from build123d import *

# Parameters (mm, degrees)
SKETCH1_R           = 37.5
SKETCH1_R_2         = 35
BOSS_EXTRUDE1_DEPTH = 40
BOSS_EXTRUDE1_TAPER = 2
CUT_EXTRUDE1_DEPTH  = 40
CIRPATTERN1_COUNT   = 10
CUT_EXTRUDE2_DEPTH  = 40
CIRPATTERN2_COUNT   = 7
CIRPATTERN2_ANGLE   = 309


with BuildPart() as part:
    # Sketch1 → Boss-Extrude1 (new body)
    with BuildSketch(Plane(origin=(0, 0, 0), x_dir=(1, 0, 0), z_dir=(0, 1, 0))):
        Circle(SKETCH1_R)
        Circle(SKETCH1_R_2, mode=Mode.SUBTRACT)
    extrude(amount=BOSS_EXTRUDE1_DEPTH, taper=BOSS_EXTRUDE1_TAPER)

    # Sketch2 → Cut-Extrude1 (cut)
    with BuildSketch(Plane(origin=(0, 0, 0), x_dir=(0, 0, -1), z_dir=(1, 0, 0))):
        with BuildLine():
            Line((-3.5, 35.795316604), (-7.534748759, 33.202081775))
            Line((-7.534748759, 33.202081775), (-4.593988586, 28.626627084))
            Line((-4.593988586, 28.626627084), (0, 25.914355347))
            Line((0, 25.914355347), (4.219955288, 28.626627084))
            Line((4.219955288, 28.626627084), (6.92128469, 33.202081775))
            Line((6.92128469, 33.202081775), (3.5, 35.795316604))
            ThreePointArc((3.5, 35.795316604), (0, 39.295316604), (-3.5, 35.795316604))
        make_face()
    cut_extrude1 = extrude(amount=-CUT_EXTRUDE1_DEPTH, mode=Mode.SUBTRACT)

    # CirPattern1: Cut-Extrude1 ×10 about axis
    cirpattern1_axis = Axis((0, 0, 0), (0, 1, 0))
    for i in range(1, CIRPATTERN1_COUNT):
        add(cut_extrude1.rotate(cirpattern1_axis, i * 360 / CIRPATTERN1_COUNT), mode=Mode.SUBTRACT)

    # Sketch3 → Cut-Extrude2 (cut)
    with BuildSketch(Plane(origin=(0, 0, 0), x_dir=(0, 0, -1), z_dir=(1, 0, 0))):
        Polygon((0, 21.378578538), (-5.541834778, 18.44293311), (0, 6.63639335), (5.541834778, 18.44293311), align=None)
    cut_extrude2 = extrude(amount=-CUT_EXTRUDE2_DEPTH, mode=Mode.SUBTRACT)

    # CirPattern2: Cut-Extrude2 ×7 about axis
    cirpattern2_axis = Axis((0, 0, 0), (0, 1, 0))
    for i in range(1, CIRPATTERN2_COUNT):
        add(cut_extrude2.rotate(cirpattern2_axis, i * CIRPATTERN2_ANGLE / (CIRPATTERN2_COUNT - 1)), mode=Mode.SUBTRACT)


solid = part.part
The model under review builds one solid part; all positions refer to its coordinate system, in mm. A direction names the side the tool comes from. Round coordinates to 2 decimals unless told otherwise and drop trailing zeros. Loops run counter-clockwise (first coordinate to the right, second up) from the corner with the lowest first, then second, coordinate; pieces in that order, holes last. Notation, with made-up numbers: (86, -1.75) -> (133, -1.75) arc R19 cw to (133, 14.25) -> close; hole circle Ø9 at (-37.5, 16). An arc over 180 degrees is marked (long way). Write item = value, one per line. Start each with the question number.
Item 1: To check wall thickness, follow L1, parallel to Z at x = 11, y = 24.5; L2, parallel to Z at x = -2, y = 6; L3, parallel to X at y = 6, z = 5.5. State the ranges of each line that lie inside material, in increasing order.
Item 2: For faces 1 (the flat face through (-20.67, 12.46, -29.87)), 2 (the flat face through (-35.78, 30.44, 5.76)), list the 3-axis set-ups (+Z, -Z, +X, -X, +Y, -Y) from which the entire face can be reached by the end or side of a thin tool; tool diameter is ignored.
Item 3: Take a section at A-A on x = 0. Give the boundary of the cut face in (y, z), plus the area to 3 significant figures.
Item 4: Mouldability with a two-part tool opening along Z and no side actions: class faces 3 (the flat face through (32.105, 30.374, -16.834)), 4 (the flat face through (-36.146, 19.931, 2.732)), 5 (the conical face through (35.3, 14.2, -11.1)), 6 (the flat face through (-32.105, 30.374, 16.834)) as released by +Z, released by -Z, zero draft, split by the parting line, or undercut.
Item 5: Insertion check: pin 1 (8 mm diameter, centred on y = 5, z = -20.5, fed in from +X); pin 2 (1 mm diameter, centred on x = 13.5, y = 24.5, fed in from +Z); pin 3 (12 mm diameter, centred on y = 28, z = -1.5, fed in from +X). Each pin has a flat end and moves straight along its axis. Give the tip position at first contact, or say it passes through.
Result:
q1.L1 = -34.95 to -34.13, 34.13 to 34.95
q1.L2 = -37.24 to -35.15, 35.15 to 37.24
q1.L3 = -36.88 to -34.78, 34.78 to 36.88
q2.face_1 = none
q2.face_2 = -X
q3.outline = (0, -37.5) -> (35.8, -36.25) -> (0, -35) -> close; (0, 35) -> (35.8, 36.25) -> (0, 37.5) -> close
q3.area = 89.5 mm²
q4.face_3 = released by -Z
q4.face_4 = undercut
q4.face_5 = split by the parting line
q4.face_6 = released by +Z
q5.pin_1 = 33.49
q5.pin_2 = 34.26
q5.pin_3 = 36.73
